Build history of the part. All positions in model axes, mm. Face numbers are marked on the shaded views. A direction names the side the tool comes from. Give positions to 0.01 mm unless a question says otherwise; leave off trailing zeros. Order: outer loops, then holes, each group sorted by start corner. A loop starts at its lowest first (then second) coordinate and runs counter-clockwise, first axis right, second up. Notation, with made-up numbers: (-16, 16) -> (19, 16) arc R11 cw to (19, 25) -> close; hole circle Ø7 at (82, 75). An arc over 180 degrees is marked (long way). One line per question, with ' | ' between items. Start each with the question number.
(1) Which spindle directions (+Z, -Z, +X, -X, +Y, -Y) get a long thin tool onto all of the face, cutting with end or side? Do the marked faces 1 and 2. Say none if no direction does.
(2) Pin check, flat tips, straight feed: pin 1 Ø3 at (y, z) = (10, -8) entering from -X; pin 2 Ø3.5 at (x, z) = (0, 0) entering from +Y; pin 3 Ø3 at (x, z) = (-0.5, -8) entering from -Y; pin 4 Ø2.5 at (x, z) = (0, 0) entering from +Y. Stop position of each tip, or through.
(3) Cut at B-B (z = 0). Give the number of separate pieces and of enclosed holes in the cut face, then the cut area to 3 significant figures.
(4) Drill centre lines: L1, parallel to X at y = 7, z = 0 (3 decimals); L2, parallel to X at y = 1.95, z = 0 (3 decimals); L3, parallel to Y at x = 35.5, z = -4.5. Where is each one in solid material? Low to high. Write a range as from..to.
(5) Cut at A-A (y = 13.75). Give the cut face in (x, z) (3 decimals), then the cut area to 3 significant figures.
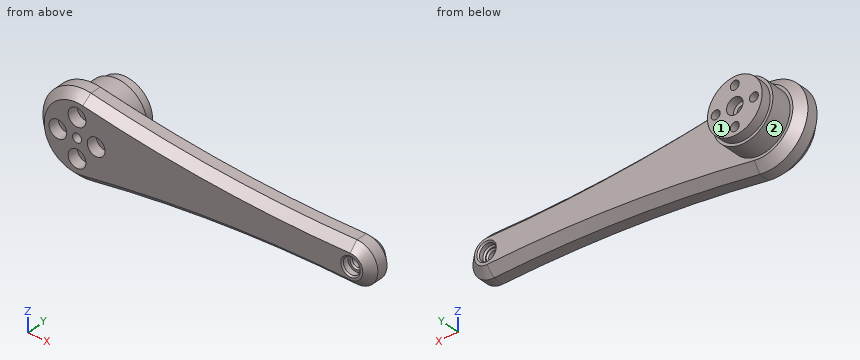
from build123d import *

# Parameters (mm, degrees)
ESQUISSE1_R                = 10
ESQUISSE1_R_2              = 1.625
BOSS_EXTRU_1_DEPTH         = 21
ESQUISSE2_R                = 3
ENL_V_MAT_EXTRU_1_DEPTH    = 3
BOSS_EXTRU_2_START         = 21
ESQUISSE3_R                = 11
ESQUISSE3_R_2              = 10
BOSS_EXTRU_2_DEPTH         = 17.5
ESQUISSE4_R                = 11
BOSS_EXTRU_3_DEPTH         = 10
ESQUISSE5_R                = 3.045
ENL_V_MAT_EXTRU_2_DEPTH    = 2.5
ESQUISSE6_R                = 1.75
ENL_V_MAT_EXTRU_3_DEPTH    = 111.106766368
CHANFREIN1_SIZE            = 3
PER_AGEAVANC_2_OUTLINE_R   = 3.25
PER_AGEAVANC_2_OUTLINE_R_2 = 1.625
PER_AGEAVANC_2_DEPTH       = 4
CHANFREIN2_SIZE            = 0.5


# Read off the part's stored shape, not the designer's step: PerçageAvancé2
with BuildPart() as part:
    # Esquisse1 → Boss.-Extru.1 (new body)
    with BuildSketch(Plane(origin=(0, 0, 0), x_dir=(1, 0, 0), z_dir=(0, 1, 0))):
        with Locations(Location((0, 0, 0), (0, 0, 90))):
            Circle(ESQUISSE1_R)
        with Locations(Location((0, 7, 0), (0, 0, 90))):
            Circle(ESQUISSE1_R_2, mode=Mode.SUBTRACT)
        with Locations(Location((7, 0, 0), (0, 0, 90))):
            Circle(ESQUISSE1_R_2, mode=Mode.SUBTRACT)
        with Locations(Location((0, -7, 0), (0, 0, 90))):
            Circle(ESQUISSE1_R_2, mode=Mode.SUBTRACT)
        with Locations(Location((-7, 0, 0), (0, 0, 90))):
            Circle(ESQUISSE1_R_2, mode=Mode.SUBTRACT)
        with Locations(Location((0, 0, 0), (0, 0, 90))):
            Circle(ESQUISSE1_R_2, mode=Mode.SUBTRACT)
    extrude(amount=BOSS_EXTRU_1_DEPTH)

    # Esquisse2 → Enlèv. mat.-Extru.1 (cut)
    with BuildSketch(Plane(origin=(0, 21, 0), x_dir=(1, 0, 0), z_dir=(0, 1, 0))):
        with Locations(Location((0, 0, 0), (0, 0, 270))):
            Circle(ESQUISSE2_R)
    extrude(amount=-ENL_V_MAT_EXTRU_1_DEPTH, mode=Mode.SUBTRACT)

    # Esquisse3 → Boss.-Extru.2 (add)
    with BuildSketch(Plane.XZ.offset(-21).offset(BOSS_EXTRU_2_START)):
        with Locations(Location((0, 0, 0), (0, 0, 90))):
            Circle(ESQUISSE3_R)
        with Locations(Location((0, 0, 0), (0, 0, 270))):
            Circle(ESQUISSE3_R_2, mode=Mode.SUBTRACT)
    extrude(amount=-BOSS_EXTRU_2_DEPTH)

    # Esquisse4 → Boss.-Extru.3 (add)
    with BuildSketch(Plane.XZ):
        with BuildLine():
            ThreePointArc((2.57876462, 14.77666989), (-15, 0), (2.57876462, -14.77666989))
            ThreePointArc((2.57876462, -14.77666989), (51.023205541, -8.75124585), (99.824833086, -7.497954158))
            ThreePointArc((99.824833086, -7.497954158), (107.5, 0), (99.824833086, 7.497954158))
            ThreePointArc((99.824833086, 7.497954158), (51.023205541, 8.75124585), (2.57876462, 14.77666989))
        make_face()
        with Locations(Location((0, 0, 0), (0, 0, 270))):
            Circle(ESQUISSE4_R, mode=Mode.SUBTRACT)
    extrude(amount=-BOSS_EXTRU_3_DEPTH)

    # Esquisse5 → Enlèv. mat.-Extru.2 (cut)
    with BuildSketch(Plane.XZ):
        with Locations(Location((100, 0, 0), (0, 0, 270))):
            Circle(ESQUISSE5_R)
    enl_v_mat_extru_2 = extrude(amount=-ENL_V_MAT_EXTRU_2_DEPTH, mode=Mode.SUBTRACT)

    # Symétrie1: Enlèv. mat.-Extru.2 across plane
    add(enl_v_mat_extru_2.mirror(Plane(origin=(0, 5, 0), x_dir=(0, 0, 1), z_dir=(0, -1, 0))), mode=Mode.SUBTRACT)

    # Esquisse6 → Enlèv. mat.-Extru.3 (cut, through all)
    with BuildSketch(Plane.XZ.offset(-2.5)):
        with Locations(Location((100, 0, 0), (0, 0, 270))):
            Circle(ESQUISSE6_R)
    extrude(amount=-ENL_V_MAT_EXTRU_3_DEPTH, mode=Mode.SUBTRACT)

    # Chanfrein1
    chanfrein1_edges = [part.edges().sort_by_distance(p)[0] for p in [
        (107.5, 10, 0),
        (51.023205541, 10, -8.75124585),
        (-15, 10, 0),
        (51.023205541, 0, 8.75124585),
        (51.023205541, 10, 8.75124585),
        (107.5, 0, 0),
        (-15, 0, 0),
        (51.023205541, 0, -8.75124585),
    ]]
    chamfer(chanfrein1_edges, length=CHANFREIN1_SIZE)

    # PerçageAvancé2 outline → PerçageAvancé2 (cut)
    # profile 1 of 4: a face of its own
    with BuildSketch(Plane(origin=(0, 0, 0), x_dir=(1, 0, 0), z_dir=(0, 1, 0))):
        with Locations((-7, 0)):
            Circle(PER_AGEAVANC_2_OUTLINE_R)
        with Locations((-7, 0)):
            Circle(PER_AGEAVANC_2_OUTLINE_R_2, mode=Mode.SUBTRACT)
    # profile 2 of 4: a face of its own
    with BuildSketch(Plane(origin=(0, 0, 0), x_dir=(1, 0, 0), z_dir=(0, 1, 0))):
        with Locations((0, 7)):
            Circle(PER_AGEAVANC_2_OUTLINE_R)
        with Locations((0, 7)):
            Circle(PER_AGEAVANC_2_OUTLINE_R_2, mode=Mode.SUBTRACT)
    # profile 3 of 4: a face of its own
    with BuildSketch(Plane(origin=(0, 0, 0), x_dir=(1, 0, 0), z_dir=(0, 1, 0))):
        with Locations((0, -7)):
            Circle(PER_AGEAVANC_2_OUTLINE_R)
        with Locations((0, -7)):
            Circle(PER_AGEAVANC_2_OUTLINE_R_2, mode=Mode.SUBTRACT)
    # profile 4 of 4: a face of its own
    with BuildSketch(Plane(origin=(0, 0, 0), x_dir=(1, 0, 0), z_dir=(0, 1, 0))):
        with Locations((7, 0)):
            Circle(PER_AGEAVANC_2_OUTLINE_R)
        with Locations((7, 0)):
            Circle(PER_AGEAVANC_2_OUTLINE_R_2, mode=Mode.SUBTRACT)
    extrude(amount=PER_AGEAVANC_2_DEPTH, mode=Mode.SUBTRACT)

    # Chanfrein2
    chanfrein2_edges = [part.edges().sort_by_distance(p)[0] for p in [
        (100, 0, 3.045),
        (100, 10, 3.045),
        (100, 7.5, 3.045),
        (100, 7.5, 1.75),
        (100, 2.5, 1.75),
    ]]
    chamfer(chanfrein2_edges, length=CHANFREIN2_SIZE)


solid = part.part
Result set:
1) face 1: +Z, -Z, +X, -X, +Y | face 2: +Y
2) pin 1: stops at x = -11.15 | pin 2: stops at y = 18 | pin 3: stops at y = 4 | pin 4: passes through
3) separate pieces: 5 | enclosed holes: 0 | area: 1,150 mm2
4) L1: x = -15..-8.625, -5.375..-1.625, 1.625..5.375, 8.625..98.25, 101.75..107.5 | L2: x = -13.95..-10.25, -3.75..-1.625, 1.625..3.75, 10.25..96.955, 103.045..106.45 | L3: y = 0..10
5) outline: circle Ø22 at (0, 0); hole circle Ø3.25 at (-7, 0); hole circle Ø3.25 at (0, -7); hole circle Ø3.25 at (0, 0); hole circle Ø3.25 at (0, 7); hole circle Ø3.25 at (7, 0) | area: 339 mm2
